from build123d import *

# Parameters (mm, degrees)
F1_DEPTH = 35.33
F2_W     = 11.5
F2_H     = 31.33
F3_DEPTH = 35
F4_W     = 10.5
F4_H     = 12
F5_DEPTH = 2


with BuildPart() as f1:
    # F0 (on Top) → F1 (new body)
    with BuildSketch(Plane.XY):
        with BuildLine():
            Line((0, 37), (0, 0))
            Line((0, 0), (15.5, 0))
            Line((15.5, 0), (15.5, 20))
            ThreePointArc((15.5, 20), (16.283103, 27.658492), (18.6, 35))
            Line((18.6, 35), (23.35, 35))
            Line((23.35, 35), (23.35, 25))
            Line((23.35, 25), (25.35, 25))
            Line((25.35, 25), (25.35, 37))
            Line((25.35, 37), (0, 37))
        make_face()
    extrude(amount=F1_DEPTH)

    # F2 (on face) → F3 (cut)
    with BuildSketch(Plane(origin=(0, 37, 0), x_dir=(-1, 0, 0), z_dir=(0, 1, 0))):
        with Locations((-7.75, 17.665)):
            Rectangle(F2_W, F2_H)
    extrude(amount=-F3_DEPTH, mode=Mode.SUBTRACT)

    # F4 (on face) → F5 (cut)
    with BuildSketch(Plane.XY.offset(35.33)):
        with Locations((7.25, 16)):
            Rectangle(F4_W, F4_H)
    extrude(amount=-F5_DEPTH, mode=Mode.SUBTRACT)


solid = f1.part
For this review, take the finished solid that the model builds, in its own axes (mm). A direction names the side the tool comes from. Round coordinates to 2 decimals unless told otherwise and drop trailing zeros. Write each loop counter-clockwise with the first axis right and the second up, starting at its lowest first coordinate (ties: lowest second). Pieces come first, ordered by that corner, then holes. Notation, with made-up numbers: (31.5, 61) - (88.5, 61) arc R23 cw to (88.5, 98) - close; hole circle Ø8 at (16, 1). An arc over 180 degrees is marked (long way). Write item = value, one per line. Start each with the question number.
1. Consider section A-A on y = 7. State the section outline as (x, z) points.
2. For pin 1 Ø10 at (y, z) = (12.5, 19.5) entering from +X; pin 2 Ø3 at (x, y) = (6.5, 13.5) entering from +Z; pin 3 Ø3.5 at (x, z) = (8, 22.5) entering from +Y, all flat-tipped, find the tip position at first contact; note any pin that passes through.
3. Consider section C-C on z = 16.5. State the section outline as (x, y) points, plus the area to 3 significant figures.
4. Wall thickness on L1, parallel to X at y = 35.5, z = 3; L2, parallel to Z at x = 13.25, y = 12.5; L3, parallel to X at y = 4.5, z = 14: over which ranges is each line inside the solid? List them lowest first.
5. Consider section D-D on y = 17.5. State the section outline as (x, z) points.
6. For faces 4 (the face through (15.5, 10, 17)), 5 (the face through (13.5, 20, 17)), 6 (the face through (16.26, 27.55, 17.42)), 7 (the face through (12.5, 16, 34)), list the 3-axis set-ups (+Z, -Z, +X, -X, +Y, -Y) from which the entire face can be reached by the end or side of a thin tool; tool diameter is ignored.
7. Consider section B-B on x = 4.25. State the section outline as (y, z) points.
8. Draft analysis for pull direction Y (two halves, no side actions). For faces 1 (the face through (7, 22, 34)), 2 (the face through (25.35, 31, 17)), 3 (the face through (21, 35, 17)), state which applies: released by +Y, released by -Y, zero draft, split by the parting line, or undercut.
Evaluation:
q1.outline = (0, 0) - (15.5, 0) - (15.5, 35.33) - (0, 35.33) - close; hole (2, 2) - (13.5, 2) - (13.5, 33.33) - (2, 33.33) - close
q2.pin_1 = 15.5
q2.pin_2 = 2
q2.pin_3 = 2
q3.outline = (0, 0) - (15.5, 0) - (15.5, 20) arc R37.84 cw to (18.6, 35) - (23.35, 35) - (23.35, 25) - (25.35, 25) - (25.35, 37) - (13.5, 37) - (13.5, 2) - (2, 2) - (2, 37) - (0, 37) - close
q3.area = 226 mm2
q4.L1 = 0 to 2, 13.5 to 25.35
q4.L2 = 0 to 2, 33.33 to 35.33
q4.L3 = 0 to 2, 13.5 to 15.5
q5.outline = (0, 0) - (15.5, 0) - (15.5, 35.33) - (12.5, 35.33) - (12.5, 33.33) - (13.5, 33.33) - (13.5, 2) - (2, 2) - (2, 35.33) - (0, 35.33) - close
q6.face_4 = +Z, -Z, +X, -Y
q6.face_5 = +Y
q6.face_6 = +Z, -Z, -Y
q6.face_7 = +Z
q7.outline = (0, 0) - (37, 0) - (37, 2) - (2, 2) - (2, 33.33) - (10, 33.33) - (10, 35.33) - (0, 35.33) - close; (22, 33.33) - (37, 33.33) - (37, 35.33) - (22, 35.33) - close
q8.face_1 = undercut
q8.face_2 = zero draft
q8.face_3 = released by -Y
